The model under review builds one solid part; all positions refer to its coordinate system, in mm. A direction names the side the tool comes from. Give positions to 0.01 mm unless a question says otherwise; leave off trailing zeros. Loops run counter-clockwise (first coordinate to the right, second up) from the corner with the lowest first, then second, coordinate; pieces in that order, holes last. Notation, with made-up numbers: (3, -24.75) - (30, -24.75) arc R12 ccw to (30, -2.75) - close; hole circle Ø5 at (-17.75, 21.25). An arc over 180 degrees is marked (long way). Return JSON: item names as keys, results as strings. Group by question number.
from build123d import *

# Parameters (mm, degrees)
SKETCH1_R           = 0.5
BOSS_EXTRUDE1_DEPTH = 1.5
SKETCH2_R           = 1.5
BOSS_EXTRUDE2_DEPTH = 12
SKETCH3_R           = 0.5
BOSS_EXTRUDE3_DEPTH = 1.5
SKETCH6_W           = 11.188914533
SKETCH6_H           = 9.773285444
CUT_EXTRUDE4_DEPTH  = 6
BOSS_EXTRUDE4_DEPTH = 2


with BuildPart() as part:
    # Sketch1 → Boss-Extrude1 (new body)
    with BuildSketch(Plane(origin=(0, 0, 0), x_dir=(1, 0, 0), z_dir=(0, 1, 0))):
        with BuildLine():
            Line((5, -1), (1.5, -1))
            Line((1.5, -1), (1.5, 2.5))
            Line((1.5, 2.5), (1.5, 3))
            ThreePointArc((1.5, 3), (0, 4.5), (-1.5, 3))
            Line((-1.5, 3), (-1.5, 2.5))
            Line((-1.5, 2.5), (-1.5, -2.5))
            ThreePointArc((-1.5, -2.5), (-1.060660172, -3.560660172), (0, -4))
            Line((0, -4), (5, -4))
            ThreePointArc((5, -4), (6.5, -2.5), (5, -1))
        make_face()
        with Locations((0, -2.5)):
            Circle(SKETCH1_R, mode=Mode.SUBTRACT)
        with BuildLine():
            Line((-0.5, 3), (-0.5, 2))
            ThreePointArc((-0.5, 2), (0, 1.5), (0.5, 2))
            Line((0.5, 2), (0.5, 3))
            ThreePointArc((0.5, 3), (0, 3.5), (-0.5, 3))
        make_face(mode=Mode.SUBTRACT)
    extrude(amount=BOSS_EXTRUDE1_DEPTH)

    # Sketch2 → Boss-Extrude2 (add)
    with BuildSketch(Plane(origin=(0, 1.5, 0), x_dir=(1, 0, 0), z_dir=(0, 1, 0))):
        with Locations((5, -2.5)):
            Circle(SKETCH2_R)
    extrude(amount=BOSS_EXTRUDE2_DEPTH)

    # Sketch3 → Boss-Extrude3 (add)
    with BuildSketch(Plane(origin=(0, 13.5, 0), x_dir=(1, 0, 0), z_dir=(0, 1, 0))):
        with BuildLine():
            Line((1.5, -1), (5, -1))
            ThreePointArc((5, -1), (6.5, -2.5), (5, -4))
            Line((5, -4), (0, -4))
            ThreePointArc((0, -4), (-1.060660172, -3.560660172), (-1.5, -2.5))
            Line((-1.5, -2.5), (-1.5, 2.5))
            Line((-1.5, 2.5), (-1.5, 3))
            ThreePointArc((-1.5, 3), (0, 4.5), (1.5, 3))
            Line((1.5, 3), (1.5, 2.5))
            Line((1.5, 2.5), (1.5, -1))
        make_face()
        with Locations((0, -2.5)):
            Circle(SKETCH3_R, mode=Mode.SUBTRACT)
        with BuildLine():
            Line((-0.5, 3), (-0.5, 2))
            ThreePointArc((-0.5, 2), (0, 1.5), (0.5, 2))
            Line((0.5, 2), (0.5, 3))
            ThreePointArc((0.5, 3), (0, 3.5), (-0.5, 3))
        make_face(mode=Mode.SUBTRACT)
    extrude(amount=BOSS_EXTRUDE3_DEPTH)

    # Sketch6 → Cut-Extrude4 (cut)
    with BuildSketch(Plane(origin=(0, 15, 0), x_dir=(1, 0, 0), z_dir=(0, 1, 0))):
        with Locations((1.642455456, 0.222776364)):
            Rectangle(SKETCH6_W, SKETCH6_H)
    extrude(amount=-CUT_EXTRUDE4_DEPTH, mode=Mode.SUBTRACT)

    # Sketch7 → Boss-Extrude4 (add)
    with BuildSketch(Plane(origin=(0, 9, 0), x_dir=(1, 0, 0), z_dir=(0, 1, 0))):
        with BuildLine():
            Line((5, -1), (5, -4))
            ThreePointArc((5, -4), (3.5, -2.5), (5, -1))
        make_face()
    extrude(amount=BOSS_EXTRUDE4_DEPTH)


solid = part.part
Item 1: Take a section at B-B (x = 4.25). State the section outline as (y, z) points.
Item 2: For P1, Ø1.1, axis at y = 1, z = -2.5, coming from the +X side; P2, Ø1, axis at x = 4.5, y = 1.5, coming from the -Z side; P3, Ø3, axis at y = 4, z = 1, coming from the -X side, all flat-tipped, find the tip position at first contact; note any pin that passes through.
Item 3: Take a section at C-C (y = 8). State the section outline as (x, z) points, then the cut area to 3 significant figures.
Item 4: Mouldability with a two-part tool opening along Z and no side actions: class faces 1 (the face through (2, 1, 4)), 2 (the face through (1.5, 1, -1)), 3 (the face through (0, 0.7, -3.5)) as +Z half, -Z half, draft (parallel to the pull), parting line (faces both ways), or undercut.
Item 5: For L1, parallel to X at y = 0.55, z = 2.5; L2, parallel to Y at x = 0.25, z = 0.5; L3, parallel to Y at x = 5.25, z = 3, list the stretches that pass through material, from the lowest coordinate up. Write a range as from..to.
Item 6: Take a section at D-D (z = 1.25). State the section outline as (x, y) points, then the cut area to 3 significant figures.
Item 7: Take a section at A-A (z = -2.25). State the section outline as (x, y) points.
Item 8: Tool access review of faces 4 (the face through (3, 1, 1)), 5 (the face through (6, 9, 2)), 6 (the face through (0.5, 0.7, -2.5)): name each direction out of +Z, -Z, +X, -X, +Y, -Y from which nothing blocks a thin tool from reaching the whole face with its end or side.
Check sheet entries:
{
 "1": {"outline": "(0, 1) - (1.5, 1) - (1.5, 1.2) - (11, 1.2) - (11, 3.8) - (1.5, 3.8) - (1.5, 4) - (0, 4) - close"},
 "2": {"P1": "stops at x = 1.5", "P2": "stops at z = 1", "P3": "stops at x = 3.5"},
 "3": {"outline": "circle Ø3 at (5, 2.5)", "area": "7.07 mm^2"},
 "4": {"face 1": "+Z half", "face 2": "draft", "face 3": "undercut"},
 "5": {"L1": "x = -1.5..-0.5, 0.5..6.5", "L2": "y = 0..1.5", "L3": "y = 0..9"},
 "6": {"outline": "(-1.5, 0) - (5.83, 0) - (5.83, 9) - (5, 9) - (5, 11) - (4.17, 11) - (4.17, 1.5) - (-1.5, 1.5) - close", "area": "25.1 mm^2"},
 "7": {"outline": "(-1.5, 0) - (-0.5, 0) - (-0.5, 1.5) - (-1.5, 1.5) - close; (0.5, 0) - (1.5, 0) - (1.5, 1.5) - (0.5, 1.5) - close"},
 "8": {"face 4": "-Z, +X, +Y, -Y", "face 5": "+Z, -Z, +X, +Y", "face 6": "+Y, -Y"}
}
